from build123d import *

# Parameters (mm, degrees)
F0_W     = 81.7405879498
F0_H     = 31.518612057
F1_DEPTH = 38.1
F2_R     = 5.08
F3_T     = -2.54


# Not quite as in the source:
# - a shell that OpenCascade refuses in one call is made with other operations: the cavity is built on its own and cut out


with BuildPart() as f1:
    # F0 (on Top) → F1 (new body, symmetric)
    with BuildSketch(Plane.XY):
        Rectangle(F0_W, F0_H)
    extrude(amount=F1_DEPTH, both=True)

    # F2
    f2_edges = [f1.edges().sort_by_distance(p)[0] for p in [
        (40.870294, -15.759306, 0),
        (0, -15.759306, 38.1),
        (-40.870294, -15.759306, 0),
        (0, -15.759306, -38.1),
        (-40.870294, 15.759306, 0),
        (-40.870294, 0, -38.1),
        (40.870294, 0, -38.1),
        (0, 15.759306, -38.1),
        (40.870294, 0, 38.1),
        (40.870294, 15.759306, 0),
        (0, 15.759306, 38.1),
        (-40.870294, 0, 38.1),
    ]]
    fillet(f2_edges, radius=F2_R)

    # F3: a shell. OpenCascade refuses it in one call, so the cavity is built on its own and cut out:
    # the body offset inwards by the wall thickness, plus a prism from it out through each open face.
    f3_core = offset(f1.part, amount=F3_T, mode=Mode.PRIVATE)
    f3_exits = [f3_core.faces().sort_by_distance(p)[0] for p in [
        (0, 13.219306, 0),
    ]]
    add(f3_core, mode=Mode.SUBTRACT)
    extrude(f3_exits, amount=-F3_T, mode=Mode.SUBTRACT)


solid = f1.part
The listing builds one solid part. Answer for the finished solid, in the listing's coordinates (mm). A direction names the side the tool comes from. Coordinates: 2 decimals unless noted, no trailing zeros. Loops run counter-clockwise (first coordinate to the right, second up) from the corner with the lowest first, then second, coordinate; pieces in that order, holes last.
1) Find section B-B on x = -19. Write down the section's boundary in (y, z).
2) Find section D-D on y = -12. Write down the section's boundary in (x, z).
3) Determine the mould class of faces 4 (the face through (0.501, 14.311, -36.572)), 5 (the face through (-37.6, 0.1, 34.8)), 6 (the face through (-39.422, 14.232, -0.462)), 7 (the face through (-35.79, 14, 0)) for opening direction Z: pulls with the +Z half, pulls with the -Z half, needs draft (parallel to the pull), parting line crosses it, or undercut.
4) Find section A-A on y = 6. Write down the section's boundary in (x, z).
5) A tool of negligible diameter and unlimited length cuts with its end or side. For faces 1 (the face through (37.6, 0.1, 34.8)), 2 (the face through (35.79, 14, 0)), 3 (the face through (-39.422, 0.15, 36.572)), from which of +Z, -Z, +X, -X, +Y, -Y can it reach the whole face along a straight path? Write none if from no direction.
6) Find the intervals of material crossed by L1, parallel to X at y = -1.5, z = -24.5; L2, parallel to Z at x = 33.5, y = 7; L3, parallel to Y at x = -23, z = 13, in increasing order.
7) Find section C-C on z = 3. Write down the section's boundary in (x, y), then the cut area to 3 significant figures.
8) Flat-ended cylindrical pins translate along their axes: pin 1 Ø3 at (x, y) = (-17, 14) entering from -Z; pin 2 Ø2 at (y, z) = (15, -1) entering from +X; pin 3 Ø1.3 at (x, y) = (14, 14) entering from +Z. Find the tip coordinate at first contact, or state that the pin passes through.
Values:
1. outline: (-15.76, -33.02) arc R5.08 ccw to (-10.68, -38.1) - (10.68, -38.1) arc R5.08 ccw to (15.76, -33.02) - (13.22, -33.02) arc R2.54 cw to (10.68, -35.56) - (-10.68, -35.56) arc R2.54 cw to (-13.22, -33.02) - (-13.22, 33.02) arc R2.54 cw to (-10.68, 35.56) - (10.68, 35.56) arc R2.54 cw to (13.22, 33.02) - (15.76, 33.02) arc R5.08 ccw to (10.68, 38.1) - (-10.68, 38.1) arc R5.08 ccw to (-15.76, 33.02) - close
2. outline: (-40.7, -33.02) arc R4.91 ccw to (-35.79, -37.93) - (35.79, -37.93) arc R4.91 ccw to (40.7, -33.02) - (40.7, 33.02) arc R4.91 ccw to (35.79, 37.93) - (-35.79, 37.93) arc R4.91 ccw to (-40.7, 33.02) - close; hole (-37.96, -33.02) arc R2.17 ccw to (-35.79, -35.19) - (35.79, -35.19) arc R2.17 ccw to (37.96, -33.02) - (37.96, 33.02) arc R2.17 ccw to (35.79, 35.19) - (-35.79, 35.19) arc R2.17 ccw to (-37.96, 33.02) - close
3. face 4: pulls with the -Z half
3. face 5: undercut
3. face 6: needs draft
3. face 7: undercut
4. outline: (-40.87, -33.02) arc R5.08 ccw to (-35.79, -38.1) - (35.79, -38.1) arc R5.08 ccw to (40.87, -33.02) - (40.87, 33.02) arc R5.08 ccw to (35.79, 38.1) - (-35.79, 38.1) arc R5.08 ccw to (-40.87, 33.02) - close; hole (-38.33, -33.02) arc R2.54 ccw to (-35.79, -35.56) - (35.79, -35.56) arc R2.54 ccw to (38.33, -33.02) - (38.33, 33.02) arc R2.54 ccw to (35.79, 35.56) - (-35.79, 35.56) arc R2.54 ccw to (-38.33, 33.02) - close
5. face 1: none
5. face 2: +Y
5. face 3: +Z, -X, +Y, -Y
6. L1: x = -40.87 to -38.33, 38.33 to 40.87
6. L2: z = -38.1 to -35.56, 35.56 to 38.1
6. L3: y = -15.76 to -13.22
7. outline: (-40.87, -10.68) arc R5.08 ccw to (-35.79, -15.76) - (35.79, -15.76) arc R5.08 ccw to (40.87, -10.68) - (40.87, 10.68) arc R5.08 ccw to (35.79, 15.76) - (35.79, 13.22) arc R2.54 cw to (38.33, 10.68) - (38.33, -10.68) arc R2.54 cw to (35.79, -13.22) - (-35.79, -13.22) arc R2.54 cw to (-38.33, -10.68) - (-38.33, 10.68) arc R2.54 cw to (-35.79, 13.22) - (-35.79, 15.76) arc R5.08 ccw to (-40.87, 10.68) - close
7. area: 351 mm2
8. pin 1: stops at z = -37.76
8. pin 2: stops at x = 39.63
8. pin 3: stops at z = 37.34
